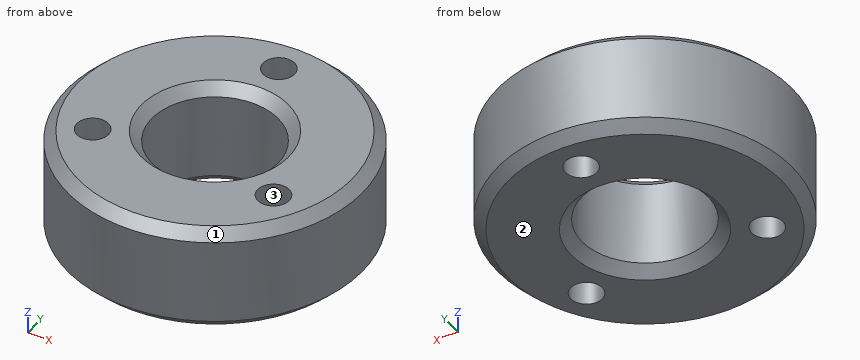
```python
from build123d import *

# Parameters (mm, degrees)
SKETCH1_R           = 14
SKETCH1_R_2         = 6
SKETCH1_R_3         = 1.5
BOSS_EXTRUDE1_DEPTH = 10
CHAMFER1_SIZE       = 1


with BuildPart() as part:
    # Sketch1 → Boss-Extrude1 (new body)
    with BuildSketch(Plane.XY):
        Circle(SKETCH1_R)
        Circle(SKETCH1_R_2, mode=Mode.SUBTRACT)
        with Locations((0, 10)):
            Circle(SKETCH1_R_3, mode=Mode.SUBTRACT)
        with Locations((8.660254038, -5)):
            Circle(SKETCH1_R_3, mode=Mode.SUBTRACT)
        with Locations((-8.660254038, -5)):
            Circle(SKETCH1_R_3, mode=Mode.SUBTRACT)
    extrude(amount=BOSS_EXTRUDE1_DEPTH)

    # Chamfer1
    chamfer1_edges = [part.edges().sort_by_distance(p)[0] for p in [
        (-14, 0, 0),
        (-14, 0, 10),
        (-6, 0, 0),
        (-6, 0, 10),
    ]]
    chamfer(chamfer1_edges, length=CHAMFER1_SIZE)


solid = part.part
```
Geometry check sheet. Reference: the model listing, model coordinates, mm. Face numbers are marked on the shaded views. Give positions to 0.01 mm unless a question says otherwise; leave off trailing zeros. Loops run counter-clockwise (first coordinate to the right, second up) from the corner with the lowest first, then second, coordinate; pieces in that order, holes last. Notation, with made-up numbers: (-29.5, 57.5) - (-18.5, 57.5) arc R36 ccw to (-18.5, 91.5) - close; hole circle Ø3 at (2.25, 27.25). An arc over 180 degrees is marked (long way). Use CSV: the item, a comma, the result in double quotes. Start each with the question number.
Q1. Section check B-B, the plane z = 7. Record the cut outline in (x, y).
Q2. Go/stop test with flat-tipped pins: pin 1 Ø1 at (y, z) = (-2, 7) entering from -X; pin 2 Ø1 at (y, z) = (10.5, 5.5) entering from -X; pin 3 Ø1 at (y, z) = (6.5, 7) entering from -X. Record where each tip stops, or that it passes through.
Q3. Section check D-D, the plane y = -5. Count the separate pieces of the cut face and the enclosed holes in it, and give its area (3 significant figures).
Q4. Section check C-C, the plane x = 0. Record the cut outline in (y, z).
Q5. Scan lines: probe 1 along Y at (x, z) = (-0.25, 5.5); probe 2 along Y at (x, z) = (-4, 1.75); probe 3 along Y at (x, z) = (-5.25, 5.25). Record each from-to range of solid material in increasing order. Write a range as from..to.
Q6. Release check for a two-part mould opening along X. For the marked faces 1, 2 and 3 record: +X half, -X half, draft (parallel to the pull), parting line (faces both ways), or undercut.
Q7. Section check A-A, the plane y = 0. Record the cut outline in (x, z).
Findings below:
1,outline,"circle Ø28 at (0, 0); hole circle Ø3 at (-8.66, -5); hole circle Ø12 at (0, 0); hole circle Ø3 at (0, 10); hole circle Ø3 at (8.66, -5)"
2,pin 1,"stops at x = -13.92"
2,pin 2,"stops at x = -9.8"
2,pin 3,"stops at x = -12.65"
3,separate pieces,"4"
3,enclosed holes,"0"
3,area,"130 mm^2"
4,outline,"(-14, 1) - (-13, 0) - (-7, 0) - (-6, 1) - (-6, 9) - (-7, 10) - (-13, 10) - (-14, 9) - close; (6, 1) - (7, 0) - (8.5, 0) - (8.5, 10) - (7, 10) - (6, 9) - close; (11.5, 0) - (13, 0) - (14, 1) - (14, 9) - (13, 10) - (11.5, 10) - close"
5,probe 1,"y = -14..-5.99, 5.99..8.52, 11.48..14"
5,probe 2,"y = -13.42..-4.47, 4.47..13.42"
5,probe 3,"y = -12.98..-2.9, 2.9..12.98"
6,face 1,"parting line"
6,face 2,"draft"
6,face 3,"undercut"
7,outline,"(-14, 1) - (-13, 0) - (-7, 0) - (-6, 1) - (-6, 9) - (-7, 10) - (-13, 10) - (-14, 9) - close; (6, 1) - (7, 0) - (13, 0) - (14, 1) - (14, 9) - (13, 10) - (7, 10) - (6, 9) - close"
